Geometry check sheet. Reference: drawing and pictorial views, mm from the part's lowest x, y, z. Give positions to 0.01 mm unless a question says otherwise; leave off trailing zeros. Write each loop counter-clockwise with the first axis right and the second up, starting at its lowest first coordinate (ties: lowest second). Pieces come first, ordered by that corner, then holes. Notation, with made-up numbers: M -18,-34 L -10,-34 A19 ccw -10,-22 Z; hole C 72,30.5 d4. An arc over 180 degrees is marked long. Answer as a JSON object with one key per item and string values.
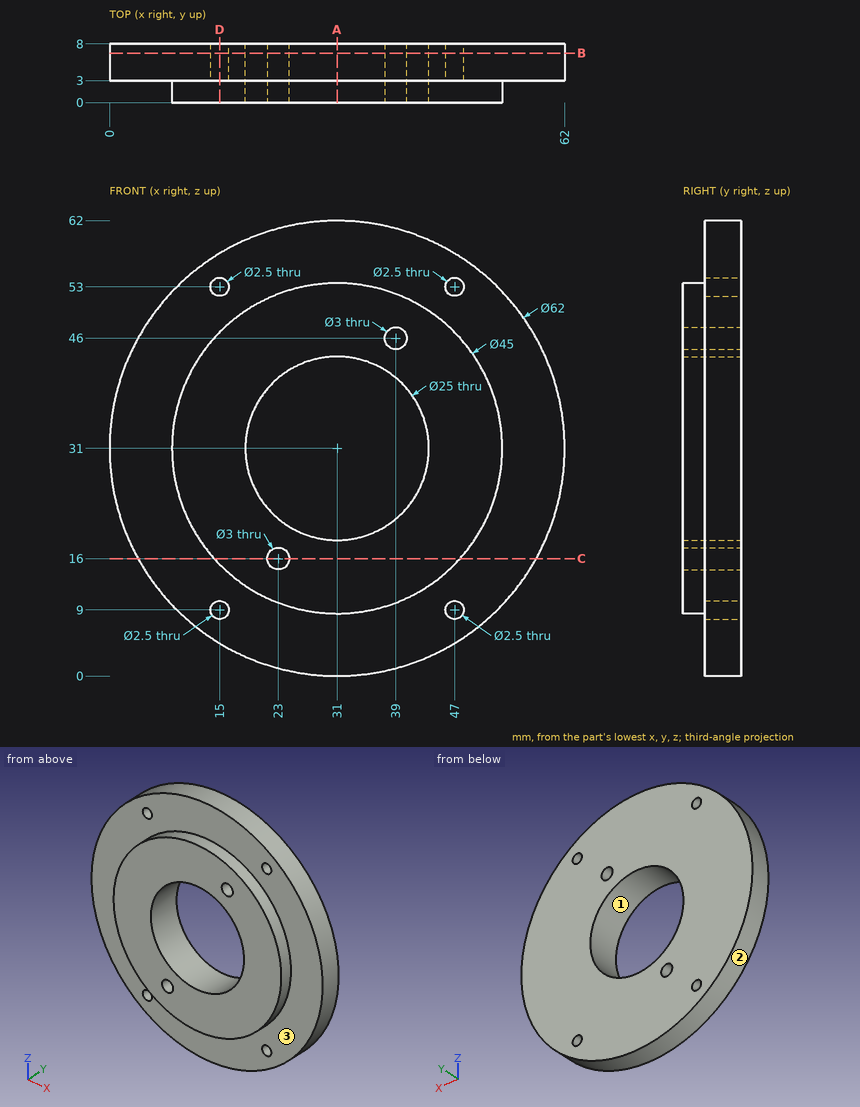
1) Section check A-A on x = 31. Record the boundary of the cut face in (y, z), and give its area (3 significant figures).
Completed:
{"outline": "M 0,8.5 L 3,8.5 L 3,0 L 8,0 L 8,18.5 L 0,18.5 Z; M 0,43.5 L 8,43.5 L 8,62 L 3,62 L 3,53.5 L 0,53.5 Z", "area": "245 mm2"}
2) Thickness scan on L1, parallel to X at y = 7.5, z = 10; L2, parallel to Z at x = 39, y = 6; L3, parallel to X at y = 5.6, z = 53. Record the ranges inside material, lowest first.
Completed:
{"L1": "x = 8.2 to 14.25, 15.75 to 46.25, 47.75 to 53.8", "L2": "z = 1.05 to 21.4, 40.6 to 44.5, 47.5 to 60.95", "L3": "x = 9.16 to 13.75, 16.25 to 45.75, 48.25 to 52.84"}
3) Go/stop test with flat-tipped pins: pin 1 (3 mm diameter, centred on x = 42.5, y = 6.5, fed in from -Z); pin 2 (2 mm diameter, centred on x = 24.5, z = 6.5, fed in from -Y). Record where each tip stops, or that it passes through.
Completed:
{"pin 1": "stops at z = 1.66", "pin 2": "stops at y = 3"}
4) Release check for a two-part mould opening along Z. For the marked faces 1, 2 and 3 record: pulls with the +Z half, pulls with the -Z half, needs draft (parallel to the pull), parting line crosses it, or undercut.
Completed:
{"face 1": "undercut", "face 2": "parting line crosses it", "face 3": "needs draft"}
5) Section check B-B on y = 6.75. Record the boundary of the cut face in (x, z), and give its area (3 significant figures).
Completed:
{"outline": "C 31,31 d62; hole C 15,9 d2.5; hole C 15,53 d2.5; hole C 31,31 d25; hole C 23,16 d3; hole C 39,46 d3; hole C 47,9 d2.5; hole C 47,53 d2.5", "area": "2,490 mm2"}
6) Section check D-D on x = 15. Record the boundary of the cut face in (y, z), and give its area (3 significant figures).
Completed:
{"outline": "M 0,15.18 L 3,15.18 L 3,10.25 L 8,10.25 L 8,51.75 L 3,51.75 L 3,46.82 L 0,46.82 Z; M 3,4.45 L 8,4.45 L 8,7.75 L 3,7.75 Z; M 3,54.25 L 8,54.25 L 8,57.55 L 3,57.55 Z", "area": "335 mm2"}
7) Section check C-C on z = 16. Record the boundary of the cut face in (x, y), and give its area (3 significant figures).
Completed:
{"outline": "M 3.87,3 L 14.23,3 L 14.23,0 L 21.5,0 L 21.5,8 L 3.87,8 Z; M 24.5,0 L 47.77,0 L 47.77,3 L 58.13,3 L 58.13,8 L 24.5,8 Z", "area": "348 mm2"}
